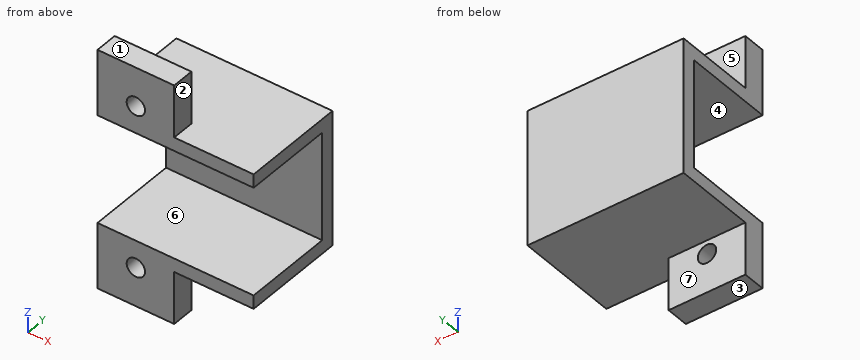
Autodesk Inventor part; units mm, degrees
ref_plane "YZ Plane" through (0, 0, 0) normal (1, 0, 0) x (0, 1, 0)
ref_plane "XZ Plane" through (0, 0, 0) normal (0, 1, 0) x (-1, 0, 0)
ref_plane "XY Plane" through (0, 0, 0) normal (0, 0, 1) x (1, 0, 0)
sketch "Sketch3" plane through (0, 0, 0) normal (1, 0, 0) x (0, 1, 0)
  line L0 (0, 0) -> (0, -7.3)
  line L1 (0, 0) -> (2.5, 0)
  line L2 (2.5, 0) -> (2.5, -5.8)
  line L3 (2.5, -5.8) -> (11.5, -5.8)
  line L4 (0, -13.3) -> (11.5, -13.3) construction
  line L5 (0, -26.6) -> (2.5, -26.6)
  line L6 (2.5, -26.6) -> (2.5, -20.8)
  line L7 (2.5, -20.8) -> (11.5, -20.8)
  line L8 (11.5, -5.8) -> (11.5, -20.8)
  line L9 (0, -7.3) -> (10, -7.3)
  line L10 (10, -7.3) -> (10, -19.3)
  line L11 (10, -19.3) -> (0, -19.3)
  line L12 (0, -19.3) -> (0, -26.6)
  dimension "d10" = 26.6
  dimension "d12" = 2.5
  dimension "d13" = 5.8
  dimension "d14" = 11.5
  dimension "d15" = 1.5
  dimension "d16" = 1.5
  dimension "d17" = 1.5
extrude "Extrusion1" add sketch "Sketch3" along normal blind 17.3
sketch "Sketch5" plane through (0, 0, -26.6) normal (0, -1, 0) x (1, 0, 0)
  line L0 (0, 0) -> (8.5, 0) construction
  line L1 (8.5, 0) -> (8.5, 5.8) construction
  line L2 (8.5, 5.8) -> (0, 5.8) construction
  line L3 (0, 5.8) -> (0, 0) construction
  line L4 (8.5, 0) -> (17.3, 0)
  line L5 (17.3, 0) -> (17.3, 5.8)
  line L6 (17.3, 5.8) -> (8.5, 5.8)
  line L7 (8.5, 5.8) -> (8.5, 0)
  line L8 (0, 19.3) -> (0, 7.3)
  line L9 (0, 13.3) -> (17.3, 13.3) construction
  line L10 (8.5, 26.6) -> (8.5, 20.8) construction
  line L11 (8.5, 26.6) -> (17.3, 26.6)
  line L12 (17.3, 26.6) -> (17.3, 20.8)
  line L13 (17.3, 20.8) -> (8.5, 20.8)
  line L14 (8.5, 20.8) -> (8.5, 26.6)
  point P0 (0, 26.6)
  dimension "d22" = 5.8
  dimension "d23" = 8.5
extrude "Extrusion2" cut sketch "Sketch5" against normal through all
sketch "Sketch6" plane through (0, 0, -7.3) normal (0, -1, 0) x (1, 0, 0)
  circle A0 centre (4.25, 3) radius 1.016
  line L0 (0, 7.3) -> (0, 0)
  line L1 (0, 0) -> (0, -12)
  line L2 (0, -6) -> (17.3, -6) construction
  line L3 (17.3, -13.5) -> (17.3, 1.5)
  circle A1 centre (4.25, -15) radius 1.016
  dimension "d26" = 2.032
  dimension "d27" = 4.25
  dimension "d28" = 18
extrude "Extrusion3" cut sketch "Sketch6" against normal through all
properties part number "gear_bracket"
The model under review builds one solid part; all positions refer to its coordinate system, in mm. Face numbers are marked on the shaded views. A direction names the side the tool comes from. Round coordinates to 2 decimals unless told otherwise and drop trailing zeros. Order: outer loops, then holes, each group sorted by start corner. A loop starts at its lowest first (then second) coordinate and runs counter-clockwise, first axis right, second up. Notation, with made-up numbers: (-36, 3.5) - (-17, 3.5) arc R25 ccw to (-17, 27.5) - close; hole circle Ø6 at (35, 26). An arc over 180 degrees is marked (long way). Answer in a Markdown table with one row per item.
(1) Machinability: for the marked faces 5, 6 and 7, which of the approach directions +Z, -Z, +X, -X, +Y, -Y give a long, thin tool a straight path to every point of the face, cutting with its end or side? Answer none if there is none.
Result set:
| item | result |
|---|---|
| face 5 | +Z, +X, -X, +Y |
| face 6 | +X, -X, -Y |
| face 7 | -Z, +X, -X, +Y |
(2) For line 1 (Z direction, x = 4.25, y = 1.35); line 2 (Z direction, x = 9.75, y = 1); line 3 (Z direction, x = 7.25, y = 1.75), list the stretches that pass through material, from the lowest coordinate up. Write a range as from..to.
Result set:
| item | result |
|---|---|
| line 1 | z = -26.6..-23.32, -21.28..-19.3, -7.3..-5.32, -3.28..0 |
| line 2 | z = -20.8..-19.3, -7.3..-5.8 |
| line 3 | z = -26.6..-19.3, -7.3..0 |
(3) Clearance check with flat-ended pins moving along their axes: P1, Ø1.2, axis at y = 0.5, z = -23.5, coming from the +X side; P2, Ø3, axis at x = 6, z = -24.5, coming from the +Y side; P3, Ø4, axis at x = 13, y = 6, coming from the -Z side; P4, Ø1.5, axis at y = 8.5, z = -17.5, coming from the -X side. State where each tip first meets the part, or that it passes through.
Result set:
| item | result |
|---|---|
| P1 | stops at x = 8.5 |
| P2 | stops at y = 2.5 |
| P3 | stops at z = -20.8 |
| P4 | passes through |
(4) Take a section at B-B on z = -22.3. Write out the cut boundary in (x, y).
Result set:
| item | result |
|---|---|
| outline | (0, 0) - (3.23, 0) - (3.23, 2.5) - (0, 2.5) - close; (5.27, 0) - (8.5, 0) - (8.5, 2.5) - (5.27, 2.5) - close |
(5) Mouldability with a two-part tool opening along Z and no side actions: class the marked faces 1, 2, 3 and 4 as released by +Z, released by -Z, zero draft, split by the parting line, or undercut.
Result set:
| item | result |
|---|---|
| face 1 | released by +Z |
| face 2 | zero draft |
| face 3 | released by -Z |
| face 4 | undercut |
(6) Take a section at D-D on y = 10.5. Write out the cut boundary in (x, z).
Result set:
| item | result |
|---|---|
| outline | (0, -20.8) - (17.3, -20.8) - (17.3, -5.8) - (0, -5.8) - close |
(7) Take a section at A-A on y = 4. Write out the cut boundary in (x, z), plus the area to 3 significant figures.
Result set:
| item | result |
|---|---|
| outline | (0, -20.8) - (17.3, -20.8) - (17.3, -19.3) - (0, -19.3) - close; (0, -7.3) - (17.3, -7.3) - (17.3, -5.8) - (0, -5.8) - close |
| area | 51.9 mm2 |
(8) Take a section at C-C on x = 13.75. Write out the cut boundary in (y, z).
Result set:
| item | result |
|---|---|
| outline | (0, -20.8) - (11.5, -20.8) - (11.5, -5.8) - (0, -5.8) - (0, -7.3) - (10, -7.3) - (10, -19.3) - (0, -19.3) - close |
